Can you work these out from the model? Positions are in its coordinate system, mm. Face numbers are marked on the shaded views. A direction names the side the tool comes from. Coordinates: 2 decimals unless noted, no trailing zeros. Order: outer loops, then holes, each group sorted by start corner. A loop starts at its lowest first (then second) coordinate and runs counter-clockwise, first axis right, second up. Notation, with made-up numbers: (73.25, -20.75) -> (116.25, -20.75) arc R10 cw to (116.25, -1.75) -> close; hole circle Ø9 at (-16.75, 49.25). An arc over 180 degrees is marked (long way). Answer as a JSON object with one key per item and string values. Group by question number.
(1) Which directions (+Z, -Z, +X, -X, +Y, -Y) give clear straight access to the entire face, cutting with the end or side of a thin tool? Please do the marked faces 1 and 2.
(2) For pin 1 (9 mm diameter, centred on x = -30, z = 0, fed in from +Y); pin 2 (7 mm diameter, centred on y = 10, z = 0, fed in from -X), each with a flat end and sliding along its axis, tell me the tip position at first contact or that it passes through.
(3) I want a section at C-C, the plane x = -30. List the corners of the cut face in (y, z) for me, plus the area to 3 significant figures.
(4) I want a section at D-D, the plane z = -3.75. List the corners of the cut face in (x, y) for me, plus the area to 3 significant figures.
(5) I want a section at B-B, the plane y = 30. List the corners of the cut face in (x, z) for me.
(6) I want a section at A-A, the plane z = 0. List the corners of the cut face in (x, y) for me.
(7) I need wall thicknesses on line 1 (Z direction, x = -2.3, y = 10); line 2 (Y direction, x = -20, z = 5.75); line 3 (X direction, y = 23, z = -6.75). Which ranges of each line are inside material? Lowest first, please.
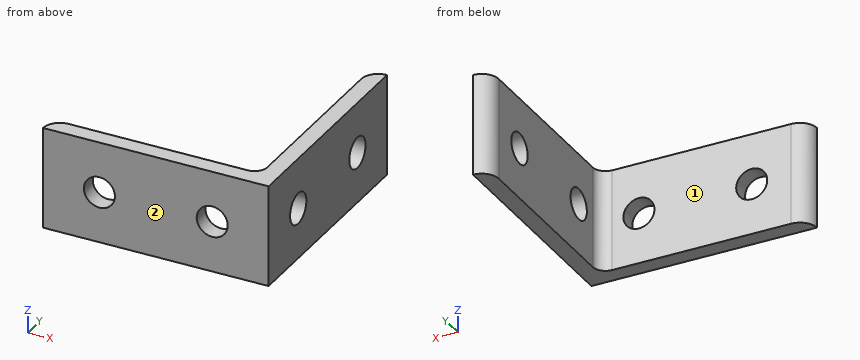
from build123d import *

# Parameters (mm, degrees)
EXTRUDE1_DEPTH     = 9
SKETCH4_R          = 2.75
CUT_EXTRUDE3_DEPTH = 56.226805086
SKETCH5_R          = 2.75
CUT_EXTRUDE4_DEPTH = 56.226805086


with BuildPart() as part:
    # Sketch1 → Extrude1 (new, symmetric)
    with BuildSketch(Plane.XY):
        with BuildLine():
            Line((0, 0), (0, 40))
            ThreePointArc((0, 40), (-2.121320344, 39.121320344), (-3, 37))
            Line((-3, 37), (-3, 5.25))
            ThreePointArc((-3, 5.25), (-3.659009742, 3.659009742), (-5.25, 3))
            Line((-5.25, 3), (-37, 3))
            ThreePointArc((-37, 3), (-39.121320344, 2.121320344), (-40, 0))
            Line((-40, 0), (0, 0))
        make_face()
    extrude(amount=EXTRUDE1_DEPTH, both=True)

    # Sketch4 → Cut-Extrude3 (cut, through all)
    with BuildSketch(Plane(origin=(0, 3, 0), x_dir=(1, 0, 0), z_dir=(0, 1, 0))):
        with Locations(Location((-10, 0, 0), (0, 0, 180))):
            Circle(SKETCH4_R)
        with Locations(Location((-30, 0, 0), (0, 0, 180))):
            Circle(SKETCH4_R)
    extrude(amount=-CUT_EXTRUDE3_DEPTH, mode=Mode.SUBTRACT)

    # Sketch5 → Cut-Extrude4 (cut, through all)
    with BuildSketch(Plane.ZY.offset(3)):
        with Locations(Location((0, 30, 0), (0, 0, 270))):
            Circle(SKETCH5_R)
        with Locations(Location((0, 10, 0), (0, 0, 270))):
            Circle(SKETCH5_R)
    extrude(amount=-CUT_EXTRUDE4_DEPTH, mode=Mode.SUBTRACT)


solid = part.part
Computed values:
{
 "1": {"face 1": "+Z, -Z, -X, +Y", "face 2": "+Z, -Z, +X, -X, -Y"},
 "2": {"pin 1": "stops at y = 3", "pin 2": "stops at x = -3"},
 "3": {"outline": "(0, -9) -> (3, -9) -> (3, -2.75) -> (0, -2.75) -> close; (0, 2.75) -> (3, 2.75) -> (3, 9) -> (0, 9) -> close", "area": "37.5 mm2"},
 "4": {"outline": "(-40, 0) -> (0, 0) -> (0, 40) arc R3 ccw to (-3, 37) -> (-3, 5.25) arc R2.25 cw to (-5.25, 3) -> (-37, 3) arc R3 ccw to start", "area": "228 mm2"},
 "5": {"outline": "(-3, -9) -> (0, -9) -> (0, -2.75) -> (-3, -2.75) -> close; (-3, 2.75) -> (0, 2.75) -> (0, 9) -> (-3, 9) -> close"},
 "6": {"outline": "(-40, 0) -> (-32.75, 0) -> (-32.75, 3) -> (-37, 3) arc R3 ccw to start; (-27.25, 0) -> (-12.75, 0) -> (-12.75, 3) -> (-27.25, 3) -> close; (-7.25, 0) -> (0, 0) -> (0, 7.25) -> (-3, 7.25) -> (-3, 5.25) arc R2.25 cw to (-5.25, 3) -> (-7.25, 3) -> close; (-3, 12.75) -> (0, 12.75) -> (0, 27.25) -> (-3, 27.25) -> close; (-3, 32.75) -> (0, 32.75) -> (0, 40) arc R3 ccw to (-3, 37) -> close"},
 "7": {"line 1": "z = -9 to -2.75, 2.75 to 9", "line 2": "y = 0 to 3", "line 3": "x = -3 to 0"}
}
